Read the model definition and answer for the solid it produces. Units are mm, in the model's axes. A direction names the side the tool comes from. Coordinates: 2 decimals unless noted, no trailing zeros. Loops run counter-clockwise (first coordinate to the right, second up) from the corner with the lowest first, then second, coordinate; pieces in that order, holes last.
Q1. Flat-ended cylindrical pins translate along their axes: P1, Ø2, axis at y = 129, z = -98, coming from the +X side; P2, Ø12, axis at x = -90, z = -60, coming from the +Y side; P3, Ø8, axis at x = -94.5, y = 124, coming from the +Z side. Find the tip coordinate at first contact, or state that the pin passes through.
Q2. Straight lines are drawn through the part: line 1 (Z direction, x = -10, y = 35.5); line 2 (X direction, y = 56, z = -104.5); line 3 (Z direction, x = -37, y = 52.5). For each, find the intervals that lie inside material, in ascending order.
Q3. Section C-C (z = -58.5) is taken. Give the vertices of the cut face in (x, y), then the cut area to 3 significant figures.
Q4. Section B-B (z = 3) is taken. Give the vertices of the cut face in (x, y).
Q5. The mould has two halves that part along Z. Classify faces 3 (the face through (-14, 0, -46)), 4 (the face through (41.006, 89.789, -106.658)), 5 (the face through (-59.36, 75.13, -151.05)): pulls with the +Z half, pulls with the -Z half, needs draft (parallel to the pull), parting line crosses it, or undercut.
Q6. Section A-A (x = -45.5) is taken. Give the vertices of the cut face in (y, z), then the cut area to 3 significant figures.
Q7. Which of the six approach directions +Z, -Z, +X, -X, +Y, -Y give full straight-line access (tool end or side, diameter ignored) to faces 1 (the face through (-35, 25.4, -68)), 2 (the face through (-49.32, 12.52, -57.32))?
Q8. Section D-D (x = -93.5) is taken. Give the vertices of the cut face in (y, z).
from build123d import *

# Parameters (mm, degrees)
F0_R     = 106.21854
F1_DEPTH = 152.4
F2_R     = 101.492892
F3_DEPTH = 127
F4_R     = 97.458229
F5_DEPTH = 127
F6_R     = 16.367238
F7_DEPTH = 25.4


with BuildPart() as f1:
    # F0 (on Front) → F1 (new body)
    with BuildSketch(Plane.XZ):
        with Locations((-36.333058, -47.356166)):
            Circle(F0_R)
    extrude(amount=-F1_DEPTH)

    # F2 (on face) → F3 (join)
    with BuildSketch(Plane.XZ):
        with Locations((-36.333058, -47.356166)):
            Circle(F2_R)
    extrude(amount=-F3_DEPTH)

    # F4 (on face) → F5 (cut)
    with BuildSketch(Plane(origin=(0, 152.4, 0), x_dir=(-1, 0, 0), z_dir=(0, 1, 0))):
        with Locations((36.333058, -47.356166)):
            Circle(F4_R)
    extrude(amount=-F5_DEPTH, mode=Mode.SUBTRACT)

    # F6 (on face) → F7 (cut)
    with BuildSketch(Plane.XZ):
        with Locations((-36.333058, -47.356166)):
            Circle(F6_R)
    extrude(amount=-F7_DEPTH, mode=Mode.SUBTRACT)


solid = f1.part
Numbers:
1. P1: stops at x = 57.57
1. P2: stops at y = 25.4
1. P3: stops at z = 44.01
2. line 1: z = -150.26 to -141.19, 46.48 to 55.55
2. line 2: x = -125.87 to -115.28, 42.61 to 53.2
2. line 3: z = -153.57 to -144.81, 50.1 to 58.86
3. outline: (-141.97, 0) - (-48.32, 0) - (-48.32, 25.4) - (-133.15, 25.4) - (-133.15, 152.4) - (-141.97, 152.4) - close; (-24.35, 0) - (69.3, 0) - (69.3, 152.4) - (60.49, 152.4) - (60.49, 25.4) - (-24.35, 25.4) - close
3. area: 7,000 mm2
4. outline: (-129.86, 0) - (57.19, 0) - (57.19, 152.4) - (47.11, 152.4) - (47.11, 25.4) - (-119.77, 25.4) - (-119.77, 152.4) - (-129.86, 152.4) - close
5. face 3: needs draft
5. face 4: undercut
5. face 5: parting line crosses it
6. outline: (0, -153.18) - (152.4, -153.18) - (152.4, -144.38) - (25.4, -144.38) - (25.4, -60.92) - (0, -60.92) - close; (0, -33.8) - (25.4, -33.8) - (25.4, 49.67) - (152.4, 49.67) - (152.4, 58.47) - (0, 58.47) - close
6. area: 6,920 mm2
7. face 1: +Y
7. face 2: +Y, -Y
8. outline: (0, -136.88) - (152.4, -136.88) - (152.4, -126.29) - (25.4, -126.29) - (25.4, 31.57) - (152.4, 31.57) - (152.4, 42.17) - (0, 42.17) - close
